Verification items for this drawing (mm, ordinates from the low corner). A direction names the side the tool comes from. Round coordinates to 2 decimals unless told otherwise and drop trailing zeros. Loops run counter-clockwise (first coordinate to the right, second up) from the corner with the lowest first, then second, coordinate; pieces in that order, holes last. Notation, with made-up numbers: (-19, 62.5) - (12, 62.5) arc R21 ccw to (12, 76.5) - close; hole circle Ø6 at (79, 13.25). An arc over 180 degrees is marked (long way). Answer in a Markdown table with one row per item. Add a question column.
(1) Access from +Z, -Z, +X, -X, +Y, -Y to the whole of each face (thin tool, end or side, straight path). Record for the marked faces 1 and 2.
(2) Thickness scan on line 1 along X through (y, z) = (1.2, 35); line 2 along Y through (x, z) = (15, 42); line 3 along X through (y, z) = (6, 41). Record the ranges inside material, lowest first.
(3) Cross-section at B-B on y = 15. Enter the section's corners in (x, z), then the cut area to 3 significant figures.
(4) Cross-section at C-C on x = 5.5. Enter the section's corners in (y, z), then the cut area to 3 significant figures.
(5) Cross-section at A-A on z = 35. Enter the section's corners in (x, y).
(6) Cross-section at D-D on z = 7. Enter the section's corners in (x, y).
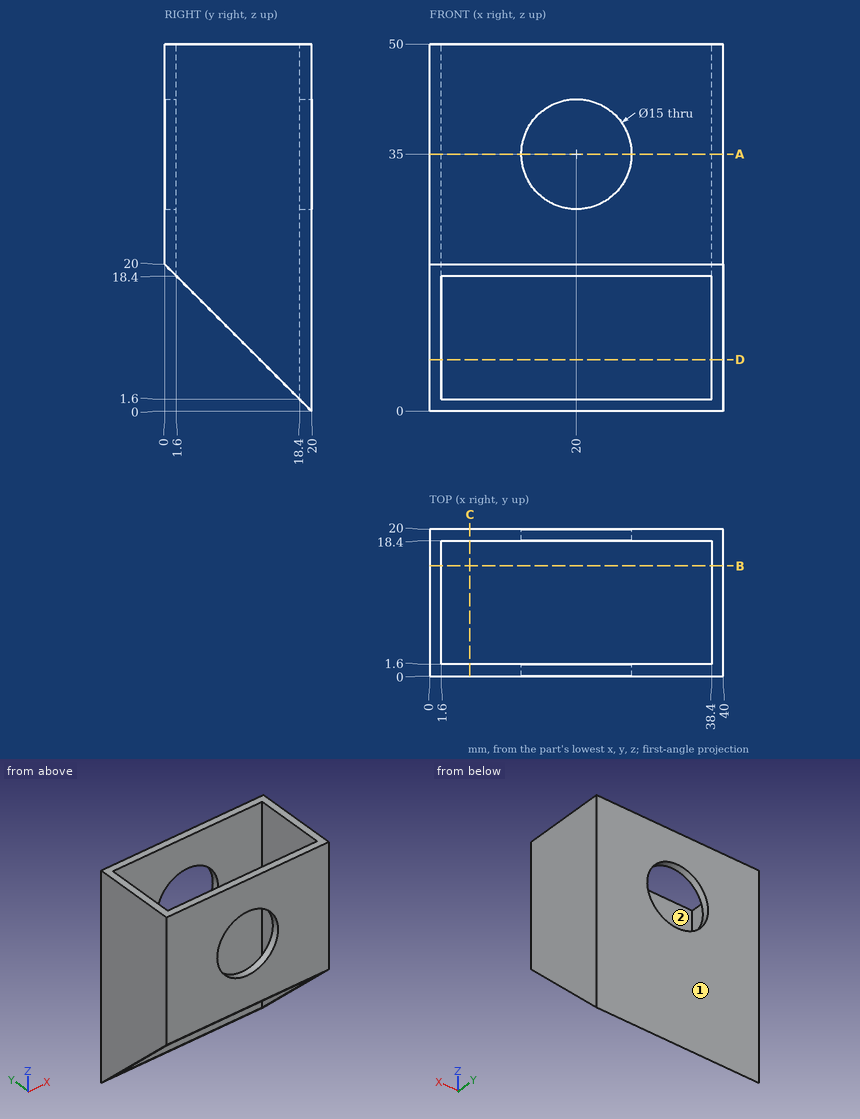
Answers:
| question | item | result |
|---|---|---|
| 1 | face 1 | +Z, -Z, +X, -X, +Y |
| 1 | face 2 | +Z, -Z |
| 2 | line 1 | x = 0 to 12.5, 27.5 to 40 |
| 2 | line 2 | y = 0 to 1.6, 18.4 to 20 |
| 2 | line 3 | x = 0 to 1.6, 38.4 to 40 |
| 3 | outline | (0, 5) - (1.6, 5) - (1.6, 50) - (0, 50) - close; (38.4, 5) - (40, 5) - (40, 50) - (38.4, 50) - close |
| 3 | area | 144 mm^2 |
| 4 | outline | (0, 20) - (1.6, 18.4) - (1.6, 50) - (0, 50) - close; (18.4, 1.6) - (20, 0) - (20, 50) - (18.4, 50) - close |
| 4 | area | 128 mm^2 |
| 5 | outline | (0, 0) - (12.5, 0) - (12.5, 1.6) - (1.6, 1.6) - (1.6, 18.4) - (12.5, 18.4) - (12.5, 20) - (0, 20) - close; (27.5, 0) - (40, 0) - (40, 20) - (27.5, 20) - (27.5, 18.4) - (38.4, 18.4) - (38.4, 1.6) - (27.5, 1.6) - close |
| 6 | outline | (0, 13) - (1.6, 13) - (1.6, 18.4) - (38.4, 18.4) - (38.4, 13) - (40, 13) - (40, 20) - (0, 20) - close |
